```python
from build123d import *

# Parameters (mm, degrees)
CROQUIS2_R              = 22.5
CROQUIS2_W              = 8
CROQUIS2_H              = 25
CROQUIS2_W_2            = 25
CROQUIS2_H_2            = 8
CROQUIS2_H_3            = 23.389278413
SALIENTE_EXTRUIR1_DEPTH = 7
CROQUIS2_4_R            = 11.1
CROQUIS2_4_R_2          = 9
SALIENTE_EXTRUIR2_DEPTH = 22
CROQUIS2_5_R            = 22.5
CROQUIS2_5_R_2          = 11.1
SALIENTE_EXTRUIR3_DEPTH = 27
CROQUIS3_R              = 1.75
CORTAR_EXTRUIR1_DEPTH   = 7
CROQUIS4_R              = 3.1
CORTAR_EXTRUIR2_DEPTH   = 2.7


with BuildPart() as part:
    # Croquis2 → Saliente-Extruir1 (new body)
    # profile 1 of 6: a face of its own
    with BuildSketch(Plane.XY):
        with BuildLine():
            Line((-5.786620614, 39.205288522), (-30.786620614, 39.205288522))
            Line((-30.786620614, 39.205288522), (-47.286620614, 39.205288522))
            Line((-47.286620614, 39.205288522), (-47.286620614, 19.816010109))
            Line((-47.286620614, 19.816010109), (-47.286620614, -5.183989891))
            Line((-47.286620614, -5.183989891), (-47.286620614, -30.183989891))
            Line((-47.286620614, -30.183989891), (-47.286620614, -49.183989891))
            ThreePointArc((-47.286620614, -49.183989891), (-45.236368082, -54.133737359), (-40.286620614, -56.183989891))
            Line((-40.286620614, -56.183989891), (-30.786620614, -56.183989891))
            Line((-30.786620614, -56.183989891), (-5.786620614, -56.183989891))
            Line((-5.786620614, -56.183989891), (3.713379386, -56.183989891))
            ThreePointArc((3.713379386, -56.183989891), (8.663126854, -54.133737359), (10.713379386, -49.183989891))
            Line((10.713379386, -49.183989891), (10.713379386, -30.183989891))
            Line((10.713379386, -30.183989891), (10.713379386, -6.794711478))
            Line((10.713379386, -6.794711478), (10.713379386, -5.183989891))
            Line((10.713379386, -5.183989891), (10.713379386, 18.205288522))
            Line((10.713379386, 18.205288522), (10.713379386, 39.205288522))
            Line((10.713379386, 39.205288522), (-5.786620614, 39.205288522))
        make_face()
        with Locations((-18.286620614, -27.183989891)):
            Circle(CROQUIS2_R, mode=Mode.SUBTRACT)
        with BuildLine():
            ThreePointArc((-29.286620614, 21.705288522), (-18.286620614, 32.705288522), (-7.286620614, 21.705288522))
            Line((-7.286620614, 21.705288522), (-7.286620614, 14.705288522))
            ThreePointArc((-7.286620614, 14.705288522), (-18.286620614, 3.705288522), (-29.286620614, 14.705288522))
            Line((-29.286620614, 14.705288522), (-29.286620614, 21.705288522))
        make_face(mode=Mode.SUBTRACT)
    # profile 2 of 6: a face of its own
    with BuildSketch(Plane.XY):
        Polygon((10.713379386, 39.205288522), (-5.786620614, 39.205288522), (-5.786620614, 48.816010109), (18.713379386, 48.816010109), (18.713379386, 18.205288522), (10.713379386, 18.205288522), align=None)
    # profile 3 of 6: a face of its own
    with BuildSketch(Plane.XY):
        Polygon((-47.286620614, 19.816010109), (-47.286620614, 39.205288522), (-30.786620614, 39.205288522), (-30.786620614, 48.816010109), (-55.286620614, 48.816010109), (-55.286620614, 19.816010109), align=None)
    # profile 4 of 6: a face of its own
    with BuildSketch(Plane.XY):
        with Locations((-51.286620614, -17.683989891)):
            Rectangle(CROQUIS2_W, CROQUIS2_H)
    # profile 5 of 6: a face of its own
    with BuildSketch(Plane.XY):
        with Locations((-18.286620614, -60.183989891)):
            Rectangle(CROQUIS2_W_2, CROQUIS2_H_2)
    # profile 6 of 6: a face of its own
    with BuildSketch(Plane.XY):
        with Locations((14.713379386, -18.489350685)):
            Rectangle(CROQUIS2_W, CROQUIS2_H_3)
    extrude(amount=SALIENTE_EXTRUIR1_DEPTH)



with BuildPart() as body_2:
    # Croquis2_4 → Saliente-Extruir2 (new body)
    with BuildSketch(Plane.XY):
        with Locations((-18.286620614, -27.183989891)):
            Circle(CROQUIS2_4_R)
        with Locations((-18.286620614, -27.183989891)):
            Circle(CROQUIS2_4_R_2, mode=Mode.SUBTRACT)
    extrude(amount=SALIENTE_EXTRUIR2_DEPTH)


with BuildPart() as part_1:
    add(part.part)

    add(body_2.part)  # Saliente-Extruir3 merges body 2
    # Croquis2_5 → Saliente-Extruir3 (add)
    with BuildSketch(Plane.XY):
        with Locations((-18.286620614, -27.183989891)):
            Circle(CROQUIS2_5_R)
        with Locations((-18.286620614, -27.183989891)):
            Circle(CROQUIS2_5_R_2, mode=Mode.SUBTRACT)
    extrude(amount=SALIENTE_EXTRUIR3_DEPTH)

    # Croquis3 → Cortar-Extruir1 (cut)
    with BuildSketch(Plane.XY.offset(7)):
        with Locations((-51.286620614, 34.316010109)):
            Circle(CROQUIS3_R)
        with Locations((-51.286620614, -17.683989891)):
            Circle(CROQUIS3_R)
        with Locations((-18.286620614, -60.183989891)):
            Circle(CROQUIS3_R)
        with Locations(Location((14.713379386, -17.683989891, 0), (0, 0, 180))):
            Circle(CROQUIS3_R)
        with Locations(Location((14.713379386, 34.316010109, 0), (0, 0, 180))):
            Circle(CROQUIS3_R)
    extrude(amount=-CORTAR_EXTRUIR1_DEPTH, mode=Mode.SUBTRACT)

    # Croquis4 → Cortar-Extruir2 (cut)
    with BuildSketch(Plane.XY.offset(7)):
        with Locations((-51.286620614, -17.683989891)):
            Circle(CROQUIS4_R)
        with Locations((-51.286620614, 34.316010109)):
            Circle(CROQUIS4_R)
        with Locations((14.713379386, 34.316010109)):
            Circle(CROQUIS4_R)
        with Locations((14.713379386, -17.683989891)):
            Circle(CROQUIS4_R)
        with Locations((-18.286620614, -60.183989891)):
            Circle(CROQUIS4_R)
    extrude(amount=-CORTAR_EXTRUIR2_DEPTH, mode=Mode.SUBTRACT)


solid = part_1.part
```
Can you work these out from the model? Positions are in its coordinate system, mm. A direction names the side the tool comes from. Coordinates: 2 decimals unless noted, no trailing zeros. Loops run counter-clockwise (first coordinate to the right, second up) from the corner with the lowest first, then second, coordinate; pieces in that order, holes last.
Item 1: Suppose I cut it at A-A (y = 41.5). Please give me the cut outline in (x, z).
Answers below:
outline: (-55.29, 0) - (-30.79, 0) - (-30.79, 7) - (-55.29, 7) - close; (-5.79, 0) - (18.71, 0) - (18.71, 7) - (-5.79, 7) - close
Item 2: If we mould it in two halves opening along Y, with no side actions, what happens to faces 1 (the face through (16, -18.87, 2.18)), 2 (the face through (-18, 39.205, 3)), 3 (the face through (-13.6, -16.9, 27))? For each: released by +Y, released by -Y, zero draft, split by the parting line, or undercut.
Answers below:
face 1: undercut
face 2: released by +Y
face 3: zero draft
Item 3: Suppose I cut it at B-B (x = -35.5). Please give me the cut outline in (y, z).
Answers below:
outline: (-56.18, 0) - (48.82, 0) - (48.82, 7) - (-12.69, 7) - (-12.69, 27) - (-41.67, 27) - (-41.67, 7) - (-56.18, 7) - close
Item 4: I'm going to push flat-ended pins straight in: pin 1 (8 mm diameter, centred on y = -17, z = 18.5, fed in from -X); pin 2 (7.5 mm diameter, centred on y = 13.5, z = 3.5, fed in from -X); pin 3 (12 mm diameter, centred on x = -34.5, z = 17.5, fed in from -Y). Where does each tip first touch, or does it pass through?
Answers below:
pin 1: stops at x = -39.92
pin 2: stops at x = -47.29
pin 3: stops at y = -47.23
Item 5: Suppose I cut it at C-C (y = 27). Please give me the cut outline in (x, z).
Answers below:
outline: (-55.29, 0) - (-27.93, 0) - (-27.93, 7) - (-55.29, 7) - close; (-8.64, 0) - (18.71, 0) - (18.71, 7) - (-8.64, 7) - close
Item 6: Suppose I cut it at D-D (z = 15.25). Please give me the cut outline in (x, y).
Answers below:
outline: circle Ø45 at (-18.29, -27.18); hole circle Ø18 at (-18.29, -27.18)
Item 7: Please list where these lines run through material, in increasing order: L1, parallel to X at y = -17.5, z = 2; L2, parallel to Z at x = -40.5, y = -41; L3, parallel to Z at x = -26.5, y = -32.
Answers below:
L1: x = -55.29 to -53.03, -49.55 to 12.97, 16.45 to 18.71
L2: z = 0 to 7
L3: z = 0 to 22
Item 8: Which directions (+Z, -Z, +X, -X, +Y, -Y) give clear straight access to the entire face, cutting with the end or side of a thin tool? Please do faces 4 (the face through (-47.287, 7, 3)), 5 (the face through (-5.787, 44, 3)), 6 (the face through (-51, -30.184, 3)), 7 (the face through (10.713, 6, 3)), 8 (the face through (-20.57, -58.09, 5.67)).
Answers below:
face 4: +Z, -Z, -X
face 5: +Z, -Z, +Y
face 6: +Z, -Z, -X, -Y
face 7: +Z, -Z, +X
face 8: +Z
